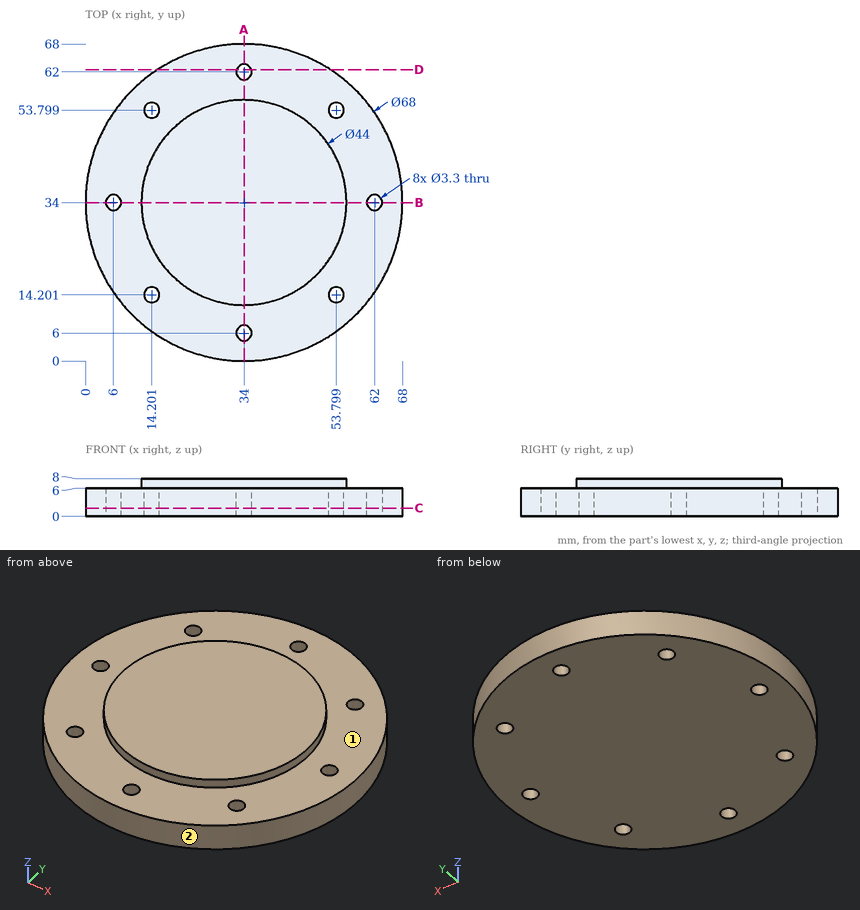
Geometry check sheet. Reference: drawing and pictorial views, mm from the part's lowest x, y, z. A direction names the side the tool comes from. Round coordinates to 2 decimals unless told otherwise and drop trailing zeros. Order: outer loops, then holes, each group sorted by start corner. A loop starts at its lowest first (then second) coordinate and runs counter-clockwise, first axis right, second up. Notation, with made-up numbers: (43, 22) - (98, 22) arc R25 cw to (98, 48) - close; hole circle Ø7 at (84, 1). An arc over 180 degrees is marked (long way). Use a Markdown table: item, result. Add a question column.
1) Gauge pin test, flat ends, axial feed: P1, Ø1.5, axis at y = 23.5, z = 7, coming from the -X side; P2, Ø4.5, axis at x = 34, y = 62, coming from the +Z side; P3, Ø1.5, axis at y = 10, z = 5.5, coming from the +X side. Record the tip position at first contact, or that the pin passes through.
2) Section check C-C (z = 1.75). Count the separate pieces of the cut face and the enclosed holes in it, then the cut area to 3 significant figures.
3) Set-up check for the marked faces 1 and 2: record each of +Z, -Z, +X, -X, +Y, -Y from which the full face is reachable in a straight line by a thin tool's end or side.
4) Section check A-A (x = 34). Record the cut outline in (y, z).
5) Section check D-D (y = 62.5). Record the cut outline in (x, z), then the cut area to 3 significant figures.
6) Thickness scan on line 1 along Y through (x, z) = (34, 3.55); line 2 along Z through (x, y) = (23, 10); line 3 along X through (y, z) = (13.5, 0.5). Record the ranges inside material, lowest first.
Established:
| question | item | result |
|---|---|---|
| 1 | P1 | x = 14.28 |
| 1 | P2 | z = 6 |
| 1 | P3 | x = 58.81 |
| 2 | separate pieces | 1 |
| 2 | enclosed holes | 8 |
| 2 | area | 3,560 mm2 |
| 3 | face 1 | +Z |
| 3 | face 2 | +Z, -Z |
| 4 | outline | (0, 0) - (4.35, 0) - (4.35, 6) - (0, 6) - close; (7.65, 0) - (60.35, 0) - (60.35, 6) - (56, 6) - (56, 8) - (12, 8) - (12, 6) - (7.65, 6) - close; (63.65, 0) - (68, 0) - (68, 6) - (63.65, 6) - close |
| 5 | outline | (15.46, 0) - (32.43, 0) - (32.43, 6) - (15.46, 6) - close; (35.57, 0) - (52.54, 0) - (52.54, 6) - (35.57, 6) - close |
| 5 | area | 204 mm2 |
| 6 | line 1 | 0 to 4.35, 7.65 to 60.35, 63.65 to 68 |
| 6 | line 2 | 0 to 6 |
| 6 | line 3 | 6.88 to 12.71, 15.69 to 52.31, 55.29 to 61.12 |
